from build123d import *

# Parameters (mm, degrees)
SKETCH_1_W             = 200
SKETCH_1_H             = 14
EXTRUDE_1_DEPTH        = 5.2
SKETCH_2_W             = 3
SKETCH_2_H             = 1
CUT_EXTRUDE_1_DEPTH    = 210
SKETCH_3_R             = 1.75
CUT_EXTRUDE_2_DEPTH    = 31
SKETCH_3_3_R           = 3
SKETCH_3_3_R_2         = 1.75
CUT_EXTRUDE_3_DEPTH    = 4.5
PATTERN_LINEAR_1_COUNT = 7
PATTERN_LINEAR_1_PITCH = 30


with BuildPart() as part:
    # 草图1 → 凸台-拉伸1 (new body)
    with BuildSketch(Plane(origin=(0, 0, 0), x_dir=(1, 0, 0), z_dir=(0, 1, 0))):
        with Locations((100, 7)):
            Rectangle(SKETCH_1_W, SKETCH_1_H)
    extrude(amount=EXTRUDE_1_DEPTH)

    # 草图2 → 切除-拉伸1 (cut)
    with BuildSketch(Plane.ZY):
        with Locations((-12.5, 3.4)):
            Rectangle(SKETCH_2_W, SKETCH_2_H)
        with Locations((-1.5, 3.4)):
            Rectangle(SKETCH_2_W, SKETCH_2_H)
    extrude(amount=-CUT_EXTRUDE_1_DEPTH, mode=Mode.SUBTRACT)

    # 草图3 → 切除-拉伸2 (cut)
    with BuildSketch(Plane(origin=(0, 5.2, 0), x_dir=(1, 0, 0), z_dir=(0, 1, 0))):
        with Locations((10, 7)):
            Circle(SKETCH_3_R)
    cut_extrude_2 = extrude(amount=-CUT_EXTRUDE_2_DEPTH, mode=Mode.SUBTRACT)

    # 草图3<3> → 切除-拉伸3 (cut)
    with BuildSketch(Plane(origin=(0, 5.2, 0), x_dir=(1, 0, 0), z_dir=(0, 1, 0))):
        with Locations((10, 7)):
            Circle(SKETCH_3_3_R)
        with Locations((10, 7)):
            Circle(SKETCH_3_3_R_2, mode=Mode.SUBTRACT)
    cut_extrude_3 = extrude(amount=-CUT_EXTRUDE_3_DEPTH, mode=Mode.SUBTRACT)

    # 阵列(线性)1: 切除-拉伸2, 切除-拉伸3 ×7
    with Locations(*[(i * PATTERN_LINEAR_1_PITCH, 0, 0) for i in range(1, PATTERN_LINEAR_1_COUNT)]):
        add(cut_extrude_2, mode=Mode.SUBTRACT)
        add(cut_extrude_3, mode=Mode.SUBTRACT)


solid = part.part
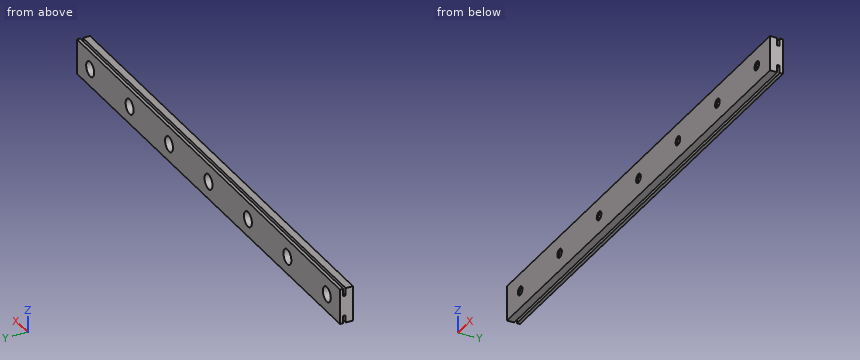
Geometry check sheet. Reference: the model listing, model coordinates, mm. Give positions to 0.01 mm unless a question says otherwise; leave off trailing zeros. Write each loop counter-clockwise with the first axis right and the second up, starting at its lowest first coordinate (ties: lowest second). Pieces come first, ordered by that corner, then holes. Notation, with made-up numbers: M -20.75,84 L 27.25,84 A24 ccw 27.25,115 Z; hole C -33.75,18 d8. An arc over 180 degrees is marked long. Answer as CSV lines item,"result". Start each with the question number.
Q1. Section check A-A, the plane y = 1.6. Record the cut outline in (x, z), then the cut area to 3 significant figures.
Q2. Section check D-D, the plane z = -7. Give the number of separate pieces and of enclosed holes in the cut face, then the cut area to 3 significant figures.
Q3. Section check C-C, the plane x = 55.5. Record the cut outline in (y, z), then the cut area to 3 significant figures.
Q4. Material ranges on L1, parallel to Y at x = 95, z = -12; L2, parallel to Y at x = 98.5, z = -8.75; L3, parallel to Z at x = 130, y = 3.45, recorded low to high.
Q5. Section check B-B, the plane x = 10. Record the cut outline in (y, z), then the cut area to 4 significant figures.
Q6. Go/stop test with a flat-tipped pin: pin 1 (3 mm diameter, centred on x = 9, z = -8, fed in from +Y). Record where the tip stops, or that it passes through.
Geometry says:
1,outline,"M 0,-14 L 200,-14 L 200,0 L 0,0 Z; hole C 10,-7 d6; hole C 40,-7 d6; hole C 70,-7 d6; hole C 100,-7 d6; hole C 130,-7 d6; hole C 160,-7 d6; hole C 190,-7 d6"
1,area,"2,600 mm^2"
2,separate pieces,"8"
2,enclosed holes,"0"
2,area,"834 mm^2"
3,outline,"M 0,-14 L 2.9,-14 L 2.9,-11 L 3.9,-11 L 3.9,-14 L 5.2,-14 L 5.2,0 L 3.9,0 L 3.9,-3 L 2.9,-3 L 2.9,0 L 0,0 Z"
3,area,"66.8 mm^2"
4,L1,"0 to 2.9, 3.9 to 5.2"
4,L2,"0 to 0.7"
4,L3,"-11 to -10, -4 to -3"
5,outline,"M 0,-14 L 2.9,-14 L 2.9,-11 L 3.9,-11 L 3.9,-14 L 5.2,-14 L 5.2,-10 L 0.7,-10 L 0.7,-8.75 L 0,-8.75 Z; M 0,-5.25 L 0.7,-5.25 L 0.7,-4 L 5.2,-4 L 5.2,0 L 3.9,0 L 3.9,-3 L 2.9,-3 L 2.9,0 L 0,0 Z"
5,area,"37.35 mm^2"
6,pin 1,"y = 0.7"
